Source: three-view drawing plus pictorial views. Frame: mm from the lowest corner of the part. A direction names the side the tool comes from. Coordinates: 2 decimals unless noted, no trailing zeros. Order: outer loops, then holes, each group sorted by start corner. A loop starts at its lowest first (then second) coordinate and runs counter-clockwise, first axis right, second up. Notation, with made-up numbers: M 69,-19.75 L 97,-19.75 A18 cw 97,-9.75 Z; hole C -12.5,-8.5 d11. An arc over 180 degrees is marked long. Use CSV: the item, a comma, the result in double quotes. Start each with the question number.
Q1. Mould query, pull axis Z, two halves, no side actions, for the marked faces 1, 2 and 3. Classes: +Z half, -Z half, draft (parallel to the pull), parting line (faces both ways), or undercut.
Q2. Section query B-B, the plane z = 8.5. Output: boundary loops of the cut face in (x, y), and give its area (3 significant figures).
Q3. Section query C-C, the plane x = 29. Output: boundary loops of the cut face in (y, z).
Q4. Section query A-A, the plane y = 0.75. Output: boundary loops of the cut face in (x, z).
Q5. Ray query, probe 1 along X at (y, z) = (1.1, 22.5); probe 2 along X at (y, z) = (3.75, 13.5); probe 3 along X at (y, z) = (3.5, 6.5). Return the intervals inside material, ascending.
Q6. First-contact query: P1, Ø1.5, axis at x = 4, z = 18.5, coming from the +Y side; P2, Ø4, axis at x = 16, z = 8.5, coming from the +Y side. Flat tips, straight axial feed; report the tip coordinate or a pass-through.
Q7. Section query D-D, the plane z = 5. Output: boundary loops of the cut face in (x, y).
Q8. Access query for the marked faces 4, 5 and 6. Directions: +Z, -Z, +X, -X, +Y, -Y. A direction counts if a zero-diameter tool reaches every point of the face in a straight line with its end or side. Return the directions, or none.
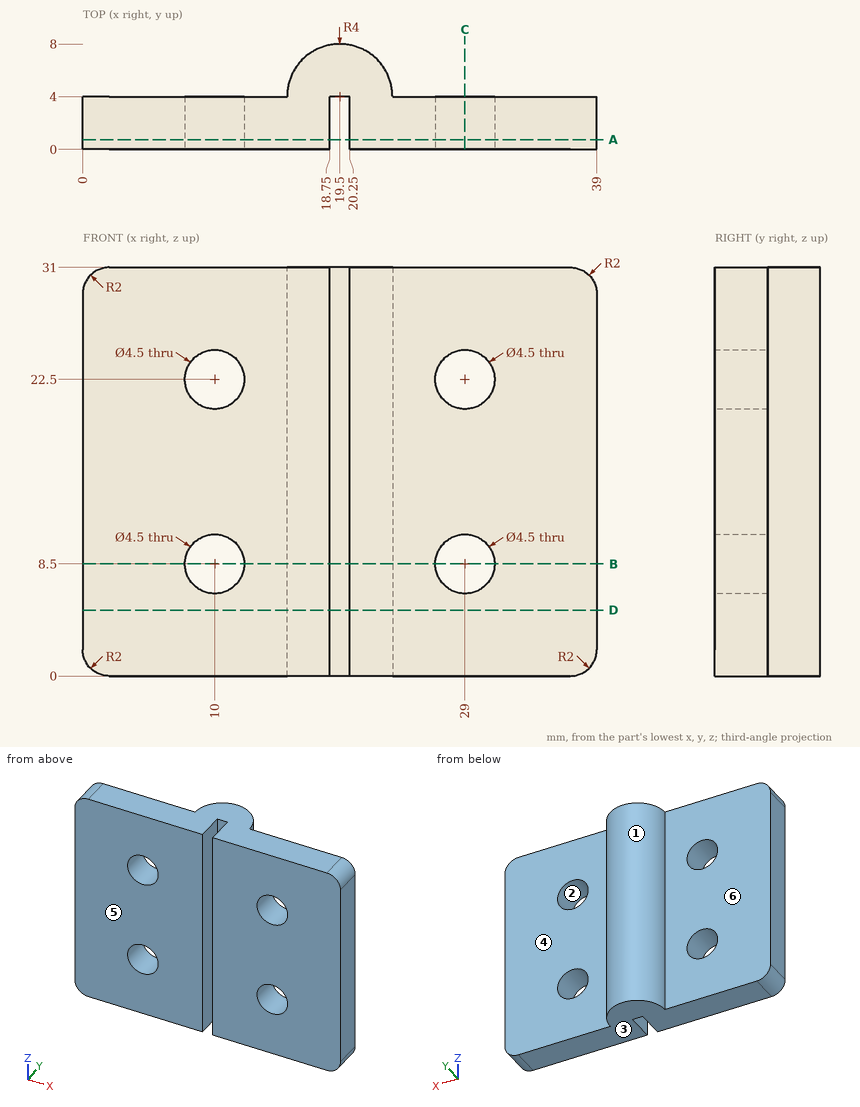
Responses:
1,face 1,"draft"
1,face 2,"undercut"
1,face 3,"-Z half"
2,outline,"M 0,0 L 7.75,0 L 7.75,4 L 0,4 Z; M 12.25,0 L 18.75,0 L 18.75,4 L 20.25,4 L 20.25,0 L 26.75,0 L 26.75,4 L 23.5,4 A4 ccw 15.5,4 L 12.25,4 Z; M 31.25,0 L 39,0 L 39,4 L 31.25,4 Z"
2,area,"139 mm²"
3,outline,"M 0,0 L 4,0 L 4,6.25 L 0,6.25 Z; M 0,10.75 L 4,10.75 L 4,20.25 L 0,20.25 Z; M 0,24.75 L 4,24.75 L 4,31 L 0,31 Z"
4,outline,"M 0,2 A2 ccw 2,0 L 18.75,0 L 18.75,31 L 2,31 A2 ccw 0,29 Z; M 20.25,0 L 37,0 A2 ccw 39,2 L 39,29 A2 ccw 37,31 L 20.25,31 Z; hole C 10,8.5 d4.5; hole C 10,22.5 d4.5; hole C 29,8.5 d4.5; hole C 29,22.5 d4.5"
5,probe 1,"x = 0 to 7.75, 12.25 to 18.75, 20.25 to 26.75, 31.25 to 39"
5,probe 2,"x = 0 to 18.75, 20.25 to 39"
5,probe 3,"x = 0 to 8.97, 11.03 to 18.75, 20.25 to 27.97, 30.03 to 39"
6,P1,"stops at y = 4"
6,P2,"stops at y = 7.71"
7,outline,"M 0,0 L 18.75,0 L 18.75,4 L 20.25,4 L 20.25,0 L 39,0 L 39,4 L 23.5,4 A4 ccw 15.5,4 L 0,4 Z"
8,face 4,"+Z, -Z, +X, +Y"
8,face 5,"+Z, -Z, +X, -X, -Y"
8,face 6,"+Z, -Z, -X, +Y"
